Read the model definition and answer for the solid it produces. Units are mm, in the model's axes. A direction names the side the tool comes from. Round coordinates to 2 decimals unless told otherwise and drop trailing zeros. Loops run counter-clockwise (first coordinate to the right, second up) from the corner with the lowest first, then second, coordinate; pieces in that order, holes last. Notation, with made-up numbers: (-30.5, 53) - (-6.5, 53) arc R5 ccw to (-6.5, 62) - close; hole circle Ø5 at (5.25, 51.5). An arc over 180 degrees is marked (long way). Answer as CSV lines item,"result".
```python
from build123d import *

# Parameters (mm, degrees)
WEB_SKETCH_W               = 58.5
WEB_SKETCH_H               = 26
WEB_DEPTH                  = 2
FLANGE_SKETCH_W            = 58.5
FLANGE_SKETCH_H            = 3.55
FLANGE_DEPTH               = 10
FLANGE_TO_TUBE_SKETCH_W    = 60.5
FLANGE_TO_TUBE_SKETCH_H    = 1.8
SERVO_CUTOUT_SKETCH_W      = 40.9
SERVO_CUTOUT_SKETCH_H      = 20.6
SERVO_CUTOUT_DEPTH         = 3
SERVO_SCREW_HOLES_SKETCH_R = 1.6
SERVO_SCREW_HOLES_DEPTH    = 3
TUBE_SCREW_HOLES_SKETCH_R  = 1.6
TUBE_SCREW_HOLES_DEPTH     = 104.05


with BuildPart() as part:
    # Web Sketch → Web (new, symmetric)
    with BuildSketch(Plane.XY):
        with Locations((-101.1, 82.5)):
            Rectangle(WEB_SKETCH_W, WEB_SKETCH_H)
    extrude(amount=WEB_DEPTH, both=True)

    # Flange Sketch → Flange (add, symmetric)
    with BuildSketch(Plane.XY):
        with Locations((-101.1, 97.275)):
            Rectangle(FLANGE_SKETCH_W, FLANGE_SKETCH_H)
    extrude(amount=FLANGE_DEPTH, both=True)

    # Flange To Tube Sketch → Flange To Tube (revolve, cut)
    with BuildSketch(Plane.XY):
        with Locations((-101.1, 100.15)):
            Rectangle(FLANGE_TO_TUBE_SKETCH_W, FLANGE_TO_TUBE_SKETCH_H)
    revolve(axis=Axis((-180.35, 0, 0), (1, 0, 0)), mode=Mode.SUBTRACT)

    # Servo Cutout Sketch → Servo Cutout (cut, symmetric)
    with BuildSketch(Plane.XY):
        with Locations((-101.1, 83.4)):
            Rectangle(SERVO_CUTOUT_SKETCH_W, SERVO_CUTOUT_SKETCH_H)
    extrude(amount=SERVO_CUTOUT_DEPTH, both=True, mode=Mode.SUBTRACT)

    # Servo Screw Holes Sketch → Servo Screw Holes (cut, symmetric)
    with BuildSketch(Plane.XY):
        with Locations((-125.85, 78.4)):
            Circle(SERVO_SCREW_HOLES_SKETCH_R)
        with Locations((-125.85, 88.4)):
            Circle(SERVO_SCREW_HOLES_SKETCH_R)
        with Locations((-76.35, 78.4)):
            Circle(SERVO_SCREW_HOLES_SKETCH_R)
        with Locations((-76.35, 88.4)):
            Circle(SERVO_SCREW_HOLES_SKETCH_R)
    extrude(amount=SERVO_SCREW_HOLES_DEPTH, both=True, mode=Mode.SUBTRACT)

    # Tube Screw Holes Sketch → Tube Screw Holes (cut, symmetric)
    with BuildSketch(Plane(origin=(0, 0, 0), x_dir=(1, 0, 0), z_dir=(0, 1, 0))):
        with Locations(Location((-125.35, -6, 0), (0, 0, 270))):
            Circle(TUBE_SCREW_HOLES_SKETCH_R)
        with Locations(Location((-125.35, 6, 0), (0, 0, 270))):
            Circle(TUBE_SCREW_HOLES_SKETCH_R)
        with Locations(Location((-76.85, -6, 0), (0, 0, 270))):
            Circle(TUBE_SCREW_HOLES_SKETCH_R)
        with Locations(Location((-76.85, 6, 0), (0, 0, 270))):
            Circle(TUBE_SCREW_HOLES_SKETCH_R)
    extrude(amount=TUBE_SCREW_HOLES_DEPTH, both=True, mode=Mode.SUBTRACT)


solid = part.part
```
1) The mould has two halves that part along X. Classify faces 1 (the face through (-102, 97, -10)), 2 (the face through (-77.6, 77.4, 0)), 3 (the face through (-130.35, 89, 0)): pulls with the +X half, pulls with the -X half, needs draft (parallel to the pull), parting line crosses it, or undercut.
Entries:
face 1,"needs draft"
face 2,"undercut"
face 3,"pulls with the -X half"
2) Find the intervals of material crossed by line 1 (Z direction, x = -76.85, y = 96.7); line 2 (Y direction, x = -125.85, z = -1); line 3 (Y direction, x = -101.5, z = -1.5), in increasing order.
Entries:
line 1,"z = -10 to -7.6, -4.4 to 4.4, 7.6 to 10"
line 2,"y = 69.5 to 76.8, 80 to 86.8, 90 to 99.05"
line 3,"y = 69.5 to 73.1, 93.7 to 99.05"
3) A cutting plane is placed at B-B, the plane x = -105. Determine the outline of the cut face in (y, z).
Entries:
outline,"(69.5, -2) - (73.1, -2) - (73.1, 2) - (69.5, 2) - close; (93.7, -2) - (95.5, -2) - (95.5, -10) - (98.74, -10) arc R99.25 ccw to (99.05, -6.3) - (99.05, 6.3) arc R99.25 ccw to (98.74, 10) - (95.5, 10) - (95.5, 2) - (93.7, 2) - close"
4) A cutting plane is placed at A-A, the plane y = 78.4. Determine the outline of the cut face in (x, z), plus the area to 3 significant figures.
Entries:
outline,"(-130.35, -2) - (-127.45, -2) - (-127.45, 2) - (-130.35, 2) - close; (-124.25, -2) - (-121.55, -2) - (-121.55, 2) - (-124.25, 2) - close; (-80.65, -2) - (-77.95, -2) - (-77.95, 2) - (-80.65, 2) - close; (-74.75, -2) - (-71.85, -2) - (-71.85, 2) - (-74.75, 2) - close"
area,"44.8 mm^2"
5) Each of these flat-tipped pins is pushed along its axis until it touches: P1, Ø6.5, axis at x = -108.5, z = 7.5, coming from the -Y side; P2, Ø3, axis at x = -76.35, y = 78.4, coming from the +Z side; P3, Ø8, axis at y = 81, z = -4, coming from the +X side; P4, Ø3.5, axis at x = -125.85, y = 78.4, coming from the -Z side. Where does it stop, or does it pass through?
Entries:
P1,"stops at y = 95.5"
P2,"passes through"
P3,"stops at x = -71.85"
P4,"stops at z = -2"
6) A cutting plane is placed at D-D, the plane x = -76.85. Determine the outline of the cut face in (y, z), plus the area to 3 significant figures.
Entries:
outline,"(69.5, -2) - (76.88, -2) - (76.88, 2) - (69.5, 2) - close; (79.92, -2) - (86.88, -2) - (86.88, 2) - (79.92, 2) - close; (89.92, -2) - (95.5, -2) - (95.5, -4.4) - (99.05, -4.4) - (99.05, 4.4) - (95.5, 4.4) - (95.5, 2) - (89.92, 2) - close; (95.5, -10) - (98.74, -10) arc R99.25 ccw to (98.96, -7.6) - (95.5, -7.6) - close; (95.5, 7.6) - (98.96, 7.6) arc R99.25 ccw to (98.74, 10) - (95.5, 10) - close"
area,"127 mm^2"
7) A tool of negligible diameter and unlimited length cuts with its end or side. For faces 4 (the face through (-71.85, 89, 0)), 5 (the face through (-80.65, 83, 0)), 6 (the face through (-102, 95.5, 6)), 7 (the face through (-102, 71, -2)), from which of +Z, -Z, +X, -X, +Y, -Y can it reach the whole face along a straight path? Write none if from no direction.
Entries:
face 4,"+Z, -Z, +X, +Y, -Y"
face 5,"+Z, -Z"
face 6,"+Z, +X, -X, -Y"
face 7,"-Z, +X, -X, -Y"
8) A cutting plane is placed at C-C, the plane z = 0. Determine the outline of the cut face in (x, y).
Entries:
outline,"(-130.35, 69.5) - (-71.85, 69.5) - (-71.85, 99.05) - (-130.35, 99.05) - close; hole circle Ø3.2 at (-125.85, 78.4); hole circle Ø3.2 at (-125.85, 88.4); hole (-121.55, 73.1) - (-80.65, 73.1) - (-80.65, 93.7) - (-121.55, 93.7) - close; hole circle Ø3.2 at (-76.35, 78.4); hole circle Ø3.2 at (-76.35, 88.4)"
